```python
from build123d import *

# Parameters (mm, degrees)
F0_W     = 1498.6
F0_H     = 1498.6
F0_R     = 574.04
F1_DEPTH = 558.8
F2_W     = 299.72
F2_H     = 299.72
F3_DEPTH = 787.4
F4_SIZE  = 38.1


with BuildPart() as f1:
    # F0 (on Front) → F1 (new body)
    with BuildSketch(Plane.XZ):
        Rectangle(F0_W, F0_H)
        Circle(F0_R, mode=Mode.SUBTRACT)
    extrude(amount=F1_DEPTH)

    # F2 (on face) → F3 (join)
    with BuildSketch(Plane.XZ.offset(558.8)):
        with Locations((-599.44, 599.44)):
            Rectangle(F2_W, F2_H)
        with Locations((-599.44, -599.44)):
            Rectangle(F2_W, F2_H)
        with Locations((599.44, -599.44)):
            Rectangle(F2_W, F2_H)
        with Locations((599.44, 599.44)):
            Rectangle(F2_W, F2_H)
    extrude(amount=F3_DEPTH)

    # F4
    f4_edges = [f1.edges().sort_by_distance(p)[0] for p in [
        (-574.04, 0, 0),
    ]]
    chamfer(f4_edges, length=F4_SIZE)


solid = f1.part
```
Check sheet for the modelled part. Datum: model origin and axes. Units: mm. A direction names the side the tool comes from. Round coordinates to 2 decimals unless told otherwise and drop trailing zeros. Loops run counter-clockwise (first coordinate to the right, second up) from the corner with the lowest first, then second, coordinate; pieces in that order, holes last. Notation, with made-up numbers: M 32.25,45 L 87.25,45 A19 ccw 87.25,81 Z; hole C 73.5,66 d7. An arc over 180 degrees is marked long. Answer as a JSON object with one key per item and string values.
1. Section check D-D (y = -84.5). Record the boundary of the cut face in (x, z), plus the area to 3 significant figures.
Reply:
{"outline": "M -749.3,-749.3 L 749.3,-749.3 L 749.3,749.3 L -749.3,749.3 Z; hole C 0,0 d1148.08", "area": "1,210,000 mm²"}
2. Section check C-C (x = 0). Record the boundary of the cut face in (y, z).
Reply:
{"outline": "M -558.8,-749.3 L 0,-749.3 L 0,-612.14 L -38.1,-574.04 L -558.8,-574.04 Z; M -558.8,574.04 L -38.1,574.04 L 0,612.14 L 0,749.3 L -558.8,749.3 Z"}
3. Section check A-A (y = -1141). Record the boundary of the cut face in (x, z).
Reply:
{"outline": "M -749.3,-749.3 L -449.58,-749.3 L -449.58,-449.58 L -749.3,-449.58 Z; M -749.3,449.58 L -449.58,449.58 L -449.58,749.3 L -749.3,749.3 Z; M 449.58,-749.3 L 749.3,-749.3 L 749.3,-449.58 L 449.58,-449.58 Z; M 449.58,449.58 L 749.3,449.58 L 749.3,749.3 L 449.58,749.3 Z"}
4. Gauge pin test, flat ends, axial feed: P1, Ø12, axis at x = 208.5, z = 536.5, coming from the -Y side; P2, Ø4, axis at x = -386.5, z = -526.5, coming from the +Y side. Record the tip position at first contact, or that the pin passes through.
Reply:
{"P1": "stops at y = -558.8", "P2": "stops at y = 0"}
5. Mould release check, pull along Z, two halves, no side actions. Record for faces 4 (the flat face through (-10, -514, -749.3)), 5 (the flat face through (-749.3, -514, -10)), 6 (the conical face through (549.805, -35.717, 173.142)): pulls with the +Z half, pulls with the -Z half, needs draft (parallel to the pull), parting line crosses it, or undercut.
Reply:
{"face 4": "pulls with the -Z half", "face 5": "needs draft", "face 6": "undercut"}
6. Access from +Z, -Z, +X, -X, +Y, -Y to the whole of each face (thin tool, end or side, straight path). Record for faces 1 (the flat face through (449.58, -947, -602)), 2 (the flat face through (-602, -947, 449.58)), 3 (the flat face through (-10, -514, 749.3)).
Reply:
{"face 1": "+Z, -Z, -Y", "face 2": "+X, -X, -Y", "face 3": "+Z, +X, -X, +Y, -Y"}
7. Section check B-B (z = 0). Record the boundary of the cut face in (x, y).
Reply:
{"outline": "M -749.3,-558.8 L -574.04,-558.8 L -574.04,-38.1 L -612.14,0 L -749.3,0 Z; M 574.04,-558.8 L 749.3,-558.8 L 749.3,0 L 612.14,0 L 574.04,-38.1 Z"}
8. Scan lines: line 1 (Z direction, x = 0, y = -405); line 2 (Z direction, x = -613, y = -1229.5). Record each from-to range of solid material in increasing order.
Reply:
{"line 1": "z = -749.3 to -574.04, 574.04 to 749.3", "line 2": "z = -749.3 to -449.58, 449.58 to 749.3"}
